Build history of the part. All positions in model axes, mm. Face numbers are marked on the shaded views. A direction names the side the tool comes from. Round coordinates to 2 decimals unless told otherwise and drop trailing zeros. Use a Markdown table: item, result. Add a question column.
Item 1: 3-axis set-ups, long thin cutter, end or side, ignore diameter. For the marked faces 1, 2, 3, 4 and 5: which of +Z, -Z, +X, -X, +Y, -Y reach the whole face in a straight line?
Item 2: Pin check, flat tips, straight feed: pin 1 (1.4 mm diameter, centred on x = 11, z = 4.5, fed in from -Y); pin 2 (1.5 mm diameter, centred on x = 37, y = -9.5, fed in from +Z); pin 3 (6 mm diameter, centred on x = 21, y = -11, fed in from +Z); pin 4 (8 mm diameter, centred on x = 40.64, y = 0, fed in from +Z) (3 decimals). Stop position of each tip, or through.
Item 3: Probe L1, parallel to Y at x = 40.64, z = -5.9; L2, parallel to Y at x = 46.5, z = 4.5; L3, parallel to Z at x = 9, y = 7. List the from-to ranges inside material, lowest first.
Item 4: Two-plate mould, pull along Y, no slides. Class the marked faces 6, 7 and 8: released by +Y, released by -Y, zero draft, split by the parting line, or undercut.
from build123d import *

# Parameters (mm, degrees)
F0_R      = 6.35
F0_R_2    = 5.08
F0_R_3    = 3.81
F1_DEPTH  = 6.35
F2_DEPTH  = 5.08
F3_DEPTH  = 3.81
F4_DEPTH  = 5.08
F5_DEPTH  = 4.445
F6_DEPTH  = 2.54
F7_DEPTH  = 3.4925
F9_W      = 25.4
F9_H      = 8.89
F10_DEPTH = 25.4


with BuildPart() as f1:
    # F0 (on Top) → F1 (new body, symmetric)
    with BuildSketch(Plane.XY):
        with BuildLine():
            ThreePointArc((20.6375, 7.9375), (15.0248399243, 5.6126600757), (12.7, 0))
            ThreePointArc((12.7, 0), (13.7452631291, -3.9371280351), (16.6057580259, -6.8373213252))
            ThreePointArc((16.6057580259, -6.8373213252), (18.5479225031, -7.657517361), (20.6375, -7.9375))
            Line((20.6375, -7.9375), (28.5891905523, -7.9375))
            Line((28.5891905523, -7.9375), (47.0239648166, -7.9375))
            add(Edge.make_bspline(
                [(47.0239648166, -7.9375), (50.1628587093, -7.9375), (54.4708534919, -7.901038248), (58.8266731571, -7.4499811863)],
                knots=[0, 0, 0, 0, 0.356398942, 0.356398942, 0.356398942, 0.356398942], degree=3))
            add(Edge.make_bspline(
                [(58.8266731571, -7.4499811863), (59.861459017, -7.3428262751), (67.7479089132, -6.3504244943), (74.9216513282, -3.7130513492), (84.8327428102, 0)],
                knots=[0.356398942, 0.356398942, 0.356398942, 0.356398942, 0.4410664934, 1, 1, 1, 1], degree=3))
            add(Edge.make_bspline(
                [(71.9619289421, 4.23150589), (75.6261537873, 3.1012059967), (79.6949939777, 1.6929446589), (84.8327428102, 0)],
                knots=[0.7129863176, 0.7129863176, 0.7129863176, 0.7129863176, 1, 1, 1, 1], degree=3))
            add(Edge.make_bspline(
                [(47.0239648166, 7.9375), (50.9085468383, 7.9375), (60.3889330239, 7.4479522989), (68.5575973368, 5.2816367669), (71.9619289421, 4.23150589)],
                knots=[0, 0, 0, 0, 0.4463297146, 0.7129863176, 0.7129863176, 0.7129863176, 0.7129863176], degree=3))
            Line((47.0239648166, 7.9375), (28.9170779288, 7.9375))
            Line((28.9170779288, 7.9375), (20.6375, 7.9375))
        make_face()
        with Locations((25.4, 0)):
            Circle(F0_R, mode=Mode.SUBTRACT)
        with Locations((40.64, 0)):
            Circle(F0_R_2, mode=Mode.SUBTRACT)
        with Locations((55.88, 0)):
            Circle(F0_R_3, mode=Mode.SUBTRACT)
    extrude(amount=F1_DEPTH, both=True)

    # F0 (on Top) → F2 (join, symmetric)
    with BuildSketch(Plane.XY):
        with BuildLine():
            ThreePointArc((4.6669778819, 8.3033091265), (8.2212708666, 4.8100239435), (9.525, 0))
            Line((9.525, 0), (12.7, 0))
            ThreePointArc((12.7, 0), (15.0248399243, 5.6126600757), (20.6375, 7.9375))
            Line((20.6375, 7.9375), (28.9170779288, 7.9375))
            Line((28.9170779288, 7.9375), (26.7881988015, 11.9220871824))
            Line((26.7881988015, 11.9220871824), (25.7645715028, 13.837993145))
            Line((25.7645715028, 13.837993145), (9.525, 13.837993145))
            Line((9.525, 13.837993145), (4.6669778819, 8.3033091265))
        make_face()
        with BuildLine():
            ThreePointArc((20.6375, -7.9375), (18.5479225031, -7.657517361), (16.6057580259, -6.8373213252))
            Line((16.6057580259, -6.8373213252), (9.525, -12.1552748606))
            Line((9.525, -12.1552748606), (11.2992681047, -14.5176804436))
            Line((11.2992681047, -14.5176804436), (31.9844596088, -14.5176804436))
            Line((31.9844596088, -14.5176804436), (31.9844596088, -12.4582387507))
            Line((31.9844596088, -12.4582387507), (28.5891905523, -7.9375))
            Line((28.5891905523, -7.9375), (20.6375, -7.9375))
        make_face()
    extrude(amount=F2_DEPTH, both=True)

    # F0 (on Top) → F3 (join, symmetric)
    with BuildSketch(Plane.XY):
        with BuildLine():
            Line((12.7, 0), (9.525, 0))
            ThreePointArc((9.525, 0), (6.7351920908, -6.7351920908), (0, -9.525))
            Line((0, -9.525), (0.9048060165, -10.7147200033))
            Line((0.9048060165, -10.7147200033), (9.525, -12.1552748606))
            Line((9.525, -12.1552748606), (16.6057580259, -6.8373213252))
            ThreePointArc((16.6057580259, -6.8373213252), (13.7452631291, -3.9371280351), (12.7, 0))
        make_face()
        with BuildLine():
            Line((47.0239648166, -7.9375), (28.5891905523, -7.9375))
            Line((28.5891905523, -7.9375), (31.9844596088, -12.4582387507))
            Line((31.9844596088, -12.4582387507), (52.2072799504, -12.4582387507))
            Line((52.2072799504, -12.4582387507), (58.8266731571, -7.4499811863))
            add(Edge.make_bspline(
                [(47.0239648166, -7.9375), (50.1628587093, -7.9375), (54.4708534919, -7.901038248), (58.8266731571, -7.4499811863)],
                knots=[0, 0, 0, 0, 0.356398942, 0.356398942, 0.356398942, 0.356398942], degree=3))
        make_face()
    extrude(amount=F3_DEPTH, both=True)

    # F0 (on Top) → F4 (join, symmetric)
    with BuildSketch(Plane.XY):
        with BuildLine():
            Line((26.7881988015, 11.9220871824), (28.9170779288, 7.9375))
            Line((28.9170779288, 7.9375), (47.0239648166, 7.9375))
            add(Edge.make_bspline(
                [(47.0239648166, 7.9375), (50.9085468383, 7.9375), (60.3889330239, 7.4479522989), (68.5575973368, 5.2816367669), (71.9619289421, 4.23150589)],
                knots=[0, 0, 0, 0, 0.4463297146, 0.7129863176, 0.7129863176, 0.7129863176, 0.7129863176], degree=3))
            Line((71.9619289421, 4.23150589), (76.4748901129, 7.6230522245))
            add(Edge.make_bspline(
                [(73.1367582265, 8.5646662812), (74.256124111, 8.2560420222), (75.365507112, 7.9395471234), (76.4748901129, 7.6230522245)],
                knots=[0.9232867166, 0.9232867166, 0.9232867166, 0.9232867166, 1, 1, 1, 1], degree=3))
            add(Edge.make_bspline(
                [(47.7164069202, 11.9794139597), (52.6527554368, 11.8770937689), (62.0717029658, 11.3991886108), (69.7025526498, 9.5115230384), (73.1367582265, 8.5646662812)],
                knots=[0.4142511087, 0.4142511087, 0.4142511087, 0.4142511087, 0.6879309771, 0.9232867166, 0.9232867166, 0.9232867166, 0.9232867166], degree=3))
            add(Edge.make_bspline(
                [(26.7881988015, 11.9220871824), (32.1440259001, 11.9989515109), (38.8226365897, 12.0947998115), (46.2365173414, 12.0100889786), (47.7164069202, 11.9794139597)],
                knots=[0, 0, 0, 0, 0.3322034202, 0.4142511087, 0.4142511087, 0.4142511087, 0.4142511087], degree=3))
        make_face()
    extrude(amount=F4_DEPTH, both=True)

    # F0 (on Top) → F5 (join, symmetric)
    with BuildSketch(Plane.XY):
        with Locations((25.4, 0)):
            Circle(F0_R)
        with Locations((40.64, 0)):
            Circle(F0_R_2)
        with Locations((55.88, 0)):
            Circle(F0_R_3)
    extrude(amount=F5_DEPTH, both=True)

    # F0 (on Top) → F6 (join, symmetric)
    with BuildSketch(Plane.XY):
        with BuildLine():
            add(Edge.make_bspline(
                [(47.7164069202, 11.9794139597), (50.2553793255, 12.9562999117), (55.1487210053, 14.6691018672), (57.5801610639, 18.6143925282), (58.7539300323, 20.4865988344)],
                knots=[0, 0, 0, 0, 0.5206708795, 1, 1, 1, 1], degree=3))
            add(Edge.make_bspline(
                [(47.7164069202, 11.9794139597), (52.6527554368, 11.8770937689), (62.0717029658, 11.3991886108), (69.7025526498, 9.5115230384), (73.1367582265, 8.5646662812)],
                knots=[0.4142511087, 0.4142511087, 0.4142511087, 0.4142511087, 0.6879309771, 0.9232867166, 0.9232867166, 0.9232867166, 0.9232867166], degree=3))
            add(Edge.make_bspline(
                [(58.7539300323, 20.4865988344), (63.4669363499, 18.1300956756), (66.2353913937, 15.6805505534), (70.7506760955, 11.9174942374), (73.1367582265, 8.5646662812)],
                knots=[0, 0, 0, 0, 0.5011324349, 1, 1, 1, 1], degree=3))
        make_face()
    extrude(amount=F6_DEPTH, both=True)

    # F0 (on Top) → F7 (join, symmetric)
    with BuildSketch(Plane.XY):
        with BuildLine():
            ThreePointArc((0, -9.525), (6.7351920908, -6.7351920908), (9.525, 0))
            ThreePointArc((9.525, 0), (8.2212708666, 4.8100239435), (4.6669778819, 8.3033091265))
            ThreePointArc((4.6669778819, 8.3033091265), (-9.2145169279, 2.4121158316), (0, -9.525))
        make_face()
    extrude(amount=F7_DEPTH, both=True)

    # F9 (on offset) → F10 (cut)
    with BuildSketch(Plane.YZ.offset(17.78)):
        with Locations((20.32, 0)):
            Rectangle(F9_W, F9_H)
    extrude(amount=F10_DEPTH, mode=Mode.SUBTRACT)


solid = f1.part
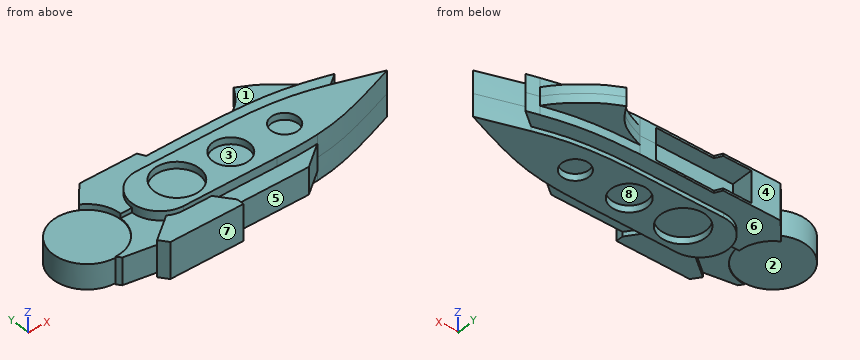
Check sheet entries:
| question | item | result |
|---|---|---|
| 1 | face 1 | +Z, +X, +Y |
| 1 | face 2 | -Z, -X |
| 1 | face 3 | +Z |
| 1 | face 4 | +Z, -Z, -X, +Y |
| 1 | face 5 | +Z, -Z, +X, -Y |
| 2 | pin 1 | y = -14.52 |
| 2 | pin 2 | z = 3.81 |
| 2 | pin 3 | z = 5.08 |
| 2 | pin 4 | z = 4.445 |
| 3 | L1 | -7.94 to -5.08, 5.08 to 7.94 |
| 3 | L2 | -7.94 to 12 |
| 3 | L3 | -5.08 to 5.08 |
| 4 | face 6 | zero draft |
| 4 | face 7 | released by -Y |
| 4 | face 8 | undercut |
